```python
from build123d import *

# Parameters (mm, degrees)
SKETCH3_W          = 215.9
SKETCH3_H          = 120.65
EXTRUDE1_DEPTH     = 4.191
SKETCH4_W          = 215.9
SKETCH4_H          = 18.415
SKETCH4_H_2        = 10.541
SKETCH4_H_3        = 7.9375
SKETCH4_H_4        = 2.032
EXTRUDE2_DEPTH     = 19.05
EXTRUDE3_DEPTH     = 17.272
SKETCH8_R          = 3.937
SKETCH8_R_2        = 1.1303
CUT_EXTRUDE1_DEPTH = 19.05


with BuildPart() as part:
    # Sketch3 → Extrude1 (new body)
    with BuildSketch(Plane.XY):
        with Locations((381, 95.25)):
            Rectangle(SKETCH3_W, SKETCH3_H)
    extrude(amount=EXTRUDE1_DEPTH)

    # Sketch4 → Extrude2 (add)
    with BuildSketch(Plane.XY):
        with Locations((381, 146.3675)):
            Rectangle(SKETCH4_W, SKETCH4_H)
        with Locations((381, 123.6345)):
            Rectangle(SKETCH4_W, SKETCH4_H_2)
        with Locations((381, 38.89375)):
            Rectangle(SKETCH4_W, SKETCH4_H_3)
        with Locations((381, 52.1335)):
            Rectangle(SKETCH4_W, SKETCH4_H_4)
    extrude(amount=EXTRUDE2_DEPTH)

    # Sketch5 → Extrude3 (add)
    with BuildSketch(Plane.XY):
        with BuildLine():
            Line((381, 58.9915), (287.3375, 58.9915))
            Line((287.3375, 58.9915), (276.225, 65.8495))
            Line((276.225, 65.8495), (279.698182312, 67.437))
            Line((279.698182312, 67.437), (290.090427682, 61.0235))
            Line((290.090427682, 61.0235), (355.6, 61.0235))
            ThreePointArc((355.6, 61.0235), (369.646316263, 64.174903412), (381.000000001, 73.025))
            ThreePointArc((381.000000001, 73.025), (392.353683737, 64.174903412), (406.4, 61.0235))
            Line((406.4, 61.0235), (471.909572318, 61.0235))
            Line((471.909572318, 61.0235), (482.301817688, 67.437))
            Line((482.301817688, 67.437), (485.775, 65.8495))
            Line((485.775, 65.8495), (474.6625, 58.9915))
            Line((474.6625, 58.9915), (381, 58.9915))
        make_face()
        Polygon((381, 87.9475), (367.3475, 87.9475), (365.125, 90.17), (367.3475, 92.3925), (381, 92.3925), (394.6525, 92.3925), (396.875, 90.17), (394.6525, 87.9475), align=None)
        with BuildLine():
            Line((436.382792366, 110.49), (325.617207634, 110.49))
            ThreePointArc((325.617207634, 110.49), (316.127546422, 108.650694601), (308.012246242, 103.399159848))
            Line((308.012246242, 103.399159848), (300.99, 96.647))
            Line((300.99, 96.647), (294.082258334, 88.9))
            Line((294.082258334, 88.9), (273.05, 109.932258334))
            Line((273.05, 109.932258334), (273.05, 112.522))
            Line((273.05, 112.522), (488.95, 112.522))
            Line((488.95, 112.522), (488.95, 109.932258334))
            Line((488.95, 109.932258334), (467.917741666, 88.9))
            Line((467.917741666, 88.9), (461.01, 96.647))
            Line((461.01, 96.647), (453.987753758, 103.399159848))
            ThreePointArc((453.987753758, 103.399159848), (445.872453578, 108.650694601), (436.382792366, 110.49))
        make_face()
    extrude(amount=EXTRUDE3_DEPTH)

    # Sketch8 → Cut-Extrude1 (cut)
    with BuildSketch(Plane.XY):
        with Locations((355.582497028, 69.847540117)):
            Circle(SKETCH8_R)
        with Locations((406.417502972, 69.847540117)):
            Circle(SKETCH8_R)
        with Locations((381, 46.99)):
            Circle(SKETCH8_R_2)
        with Locations((460.95285, 46.99)):
            Circle(SKETCH8_R_2)
        with Locations((301.04715, 46.99)):
            Circle(SKETCH8_R_2)
        with BuildLine():
            ThreePointArc((319.409826978, 89.545574531), (322.509420435, 94.391866743), (326.25811196, 98.755505093))
            ThreePointArc((326.25811196, 98.755505093), (326.161980776, 101.078429217), (323.852023449, 100.815152101))
            ThreePointArc((323.852023449, 100.815152101), (319.896382713, 96.191952728), (316.621455618, 91.063998107))
            ThreePointArc((316.621455618, 91.063998107), (317.25642951, 88.910600639), (319.409826978, 89.545574531))
        make_face()
        with BuildLine():
            ThreePointArc((438.147976551, 100.815152101), (442.103617287, 96.191952728), (445.378544382, 91.063998107))
            ThreePointArc((445.378544382, 91.063998107), (444.74357049, 88.910600639), (442.590173022, 89.545574531))
            ThreePointArc((442.590173022, 89.545574531), (439.490579565, 94.391866743), (435.74188804, 98.755505093))
            ThreePointArc((435.74188804, 98.755505093), (435.838019224, 101.078429217), (438.147976551, 100.815152101))
        make_face()
    extrude(amount=CUT_EXTRUDE1_DEPTH, mode=Mode.SUBTRACT)


solid = part.part
```
The model under review builds one solid part; all positions refer to its coordinate system, in mm. A direction names the side the tool comes from. Coordinates: 2 decimals unless noted, no trailing zeros. Write each loop counter-clockwise with the first axis right and the second up, starting at its lowest first coordinate (ties: lowest second). Pieces come first, ordered by that corner, then holes.
1) We need section C-C on y = 107. State the section outline as (x, z) points.
2) Clearance check with flat-ended pins moving along their axes: pin 1 Ø6 at (x, y) = (450, 47) entering from +Z; pin 2 Ø19 at (x, y) = (391.5, 106) entering from +Z; pin 3 Ø5 at (y, z) = (93.5, 14) entering from -X; pin 4 Ø6.5 at (x, y) = (406.42, 69.85) entering from -Z. State where each tip first meets the part, or that it passes through.
3) We need section A-A on z = 15. Count the separate pieces of the cut face and the enclosed holes in it, then the cut area to 3 significant figures.
4) The part is to be moulded in two halves that separate along Y. For faces 1 (the face through (273.05, 94, 3)), 2 (the face through (379, 42.862, 12)), say which applies: pulls with the +Y half, pulls with the -Y half, needs draft (parallel to the pull), parting line crosses it, or undercut.
5) Machinability: for faces 3 (the face through (283.71, 99.27, 10.64)), 4 (the face through (379, 137.16, 12)), 5 (the face through (381, 92.392, 11)), which of the approach directions +Z, -Z, +X, -X, +Y, -Y give a long, thin tool a straight path to every point of the face, cutting with its end or side? Answer none if there is none.
6) To check wall thickness, follow probe 1 along X at (y, z) = (46.99, 1.5); probe 2 along Y at (x, z) = (430.5, 13) (1 decimal); probe 3 along Y at (x, z) = (283.5, 17.5) (1 decimal). State the ranges of each line that lie inside material, in increasing order.
Answer list:
1. outline: (273.05, 0) - (488.95, 0) - (488.95, 4.19) - (486.02, 4.19) - (486.02, 17.27) - (449.23, 17.27) - (449.23, 4.19) - (312.77, 4.19) - (312.77, 17.27) - (275.98, 17.27) - (275.98, 4.19) - (273.05, 4.19) - close
2. pin 1: stops at z = 4.19
2. pin 2: stops at z = 17.27
2. pin 3: stops at x = 286.98
2. pin 4: passes through
3. separate pieces: 7
3. enclosed holes: 0
3. area: 10,600 mm2
4. face 1: needs draft
4. face 2: undercut
5. face 3: +Z, -X
5. face 4: +Z, +X, -X
5. face 5: +Z
6. probe 1: x = 273.05 to 299.92, 302.18 to 379.87, 382.13 to 459.82, 462.08 to 488.95
6. probe 2: y = 34.9 to 42.9, 51.1 to 53.1, 59 to 61, 110.5 to 112.5, 118.4 to 128.9, 137.2 to 155.6
6. probe 3: y = 34.9 to 42.9, 51.1 to 53.1, 118.4 to 128.9, 137.2 to 155.6
